Can you work these out from the model? Positions are in its coordinate system, mm. Face numbers are marked on the shaded views. Round coordinates to 2 decimals unless told otherwise and drop trailing zeros. Write each loop counter-clockwise with the first axis right and the second up, starting at its lowest first coordinate (ties: lowest second). Pieces come first, ordered by that corner, then holes.
Q1. If we section it at C-C (y = 3): Please give me the cut outline in (x, z), plus the area to 3 significant figures.
Q2. If we section it at B-B (y = 8.5): Please give me the cut outline in (x, z).
Q3. Please list where these lines run through material, in increasing order: line 1 along Y through (x, z) = (1.5, 0); line 2 along Y through (x, z) = (3.4, 0); line 3 along Y through (x, z) = (4.25, -2).
Q4. If we section it at D-D (y = -6.5): Please give me the cut outline in (x, z), plus the area to 3 significant figures.
Q5. I'm going to push flat-ended pins straight in: pin 1 Ø2 at (x, y) = (1.5, -6.5) entering from -Z; pin 2 Ø3 at (y, z) = (3, -3) entering from +X; pin 3 Ø2 at (x, y) = (1, -3) entering from +Z. Where does each tip first touch, or does it pass through?
Q6. We'd pull the mould along Y, two halves only. Please class the marked faces 1, 2 and 3: +Y half, -Y half, draft (parallel to the pull), parting line (faces both ways), or undercut.
Q7. If we section it at A-A (z = 0): Please give me the cut outline in (x, y) (3 decimals), plus the area to 3 significant figures.
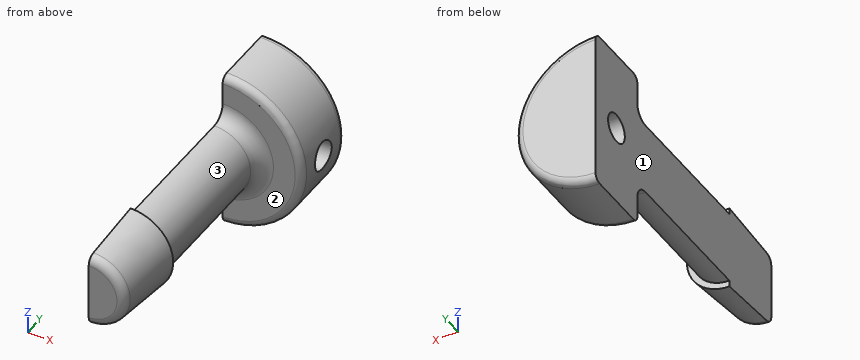
from build123d import *

# Parameters (mm, degrees)
REVOLUTION001_ANGLE = 180
FILLET003_R         = 0.6
FILLET004_R         = 1
FILLET005_R         = 0.5
SKETCH001_R         = 1
POCKET_DEPTH        = 0.001
POCKET_DEPTH_BACK   = 5.501


with BuildPart() as part:
    # Sketch002 → Revolution001 (revolve)
    with BuildSketch(Plane.YZ):
        Polygon((-10.5, 2.5), (-5.5, 2.935), (-5.5, 2.5), (5.5, 2.5), (5.5, 5.5), (10.5, 5.5), (10.5, 0), (-10.5, 0), align=None)
    revolve(axis=Axis((0, 0, 0), (0, 1, 0)), revolution_arc=REVOLUTION001_ANGLE)

    # Fillet003
    fillet003_edges = [part.edges().sort_by_distance(p)[0] for p in [
        (2.5, -10.5, 0),
    ]]
    fillet(fillet003_edges, radius=FILLET003_R)

    # Fillet004
    fillet004_edges = [part.edges().sort_by_distance(p)[0] for p in [
        (2.5, 5.5, 0),
    ]]
    fillet(fillet004_edges, radius=FILLET004_R)

    # Fillet005
    fillet005_edges = [part.edges().sort_by_distance(p)[0] for p in [
        (5.5, 5.5, 0),
        (5.5, 10.5, 0),
    ]]
    fillet(fillet005_edges, radius=FILLET005_R)

    # Sketch001 → Pocket (cut, two sides)
    with BuildSketch(Plane.YZ) as pocket_sk:
        with Locations((8, 0)):
            Circle(SKETCH001_R)
    extrude(amount=-POCKET_DEPTH, mode=Mode.SUBTRACT)
    extrude(pocket_sk.sketch, amount=POCKET_DEPTH_BACK, mode=Mode.SUBTRACT)


solid = part.part
A:
1. outline: (0, -2.5) arc R2.5 ccw to (0, 2.5) - close
1. area: 9.82 mm2
2. outline: (0, -5.5) arc R5.5 ccw to (5.43, -0.87) - (0, -0.87) - close; (0, 0.87) - (5.43, 0.87) arc R5.5 ccw to (0, 5.5) - close
3. line 1: y = -10.5 to 7, 9 to 10.5
3. line 2: y = 5.49 to 7, 9 to 10.5
3. line 3: y = 5.5 to 10.5
4. outline: (0, -2.85) arc R2.85 ccw to (0, 2.85) - close
4. area: 12.7 mm2
5. pin 1: stops at z = -2.82
5. pin 2: stops at x = 2
5. pin 3: stops at z = 2.5
6. face 1: draft
6. face 2: -Y half
6. face 3: undercut
7. outline: (0, -10.5) - (1.95, -10.5) arc R0.6 ccw to (2.548, -9.952) - (2.935, -5.5) - (2.5, -5.5) - (2.5, 4.5) arc R1 cw to (3.5, 5.5) - (5, 5.5) arc R0.5 ccw to (5.5, 6) - (5.5, 7) - (0, 7) - close; (0, 9) - (5.5, 9) - (5.5, 10) arc R0.5 ccw to (5, 10.5) - (0, 10.5) - close
7. area: 57.6 mm2
